The listing builds one solid part. Answer for the finished solid, in the listing's coordinates (mm). Face numbers are marked on the shaded views. Coordinates: 2 decimals unless noted, no trailing zeros. Order: outer loops, then holes, each group sorted by start corner. A loop starts at its lowest first (then second) coordinate and runs counter-clockwise, first axis right, second up. Notation, with made-up numbers: (-17.75, -36.75) -> (40.25, -36.75) arc R26 ccw to (40.25, -22.75) -> close; hole circle Ø6 at (83, 20.5). An arc over 180 degrees is marked (long way). One line per question, with ' | ' between items.
from build123d import *


# Read off the part's stored shape, not the designer's step: 抽壳1
with BuildPart() as part:
    # 草图1 → 旋转1 (revolve)
    with BuildSketch(Plane.XY, mode=Mode.PRIVATE) as revolve_1_sk:
        with BuildLine():
            Line((0, 0), (32, 0))
            Line((32, 0), (32, 2))
            Line((32, 2), (35, 2))
            Line((35, 2), (35, 5))
            Line((35, 5), (32, 5))
            Line((32, 5), (32, 7))
            Line((32, 7), (6, 12))
            Line((6, 12), (6, 15))
            ThreePointArc((6, 15), (9.486832981, 26.16227766), (0, 33))
            Line((0, 33), (0, 0))
        make_face()
    revolve(revolve_1_sk.sketch.rotate(Axis((0, 0, 0), (0, 1, 0)), 90), axis=Axis((0, 0, 0), (0, 1, 0)))

    # 抽壳1 outline → 抽壳1 (revolve, cut)
    with BuildSketch(Plane.XY):
        Polygon((29, 0), (29, 4.521953317), (0, 10.098876393), (0, 0), align=None)
    revolve(axis=Axis((0, 0, 0), (0, 1, 0)), mode=Mode.SUBTRACT)


solid = part.part
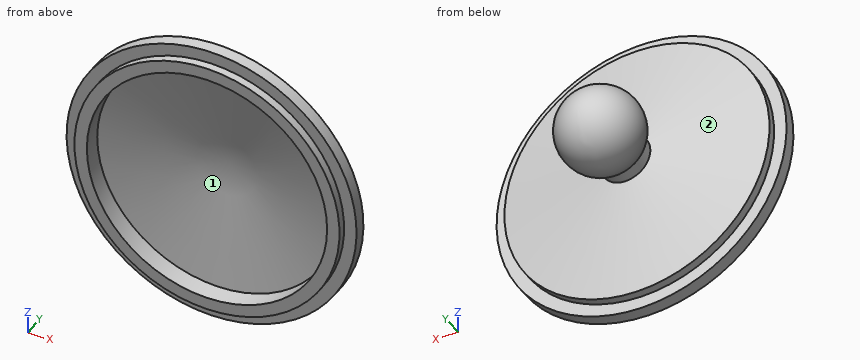
Item 1: Section B-B, the plane y = 13 is taken. Give the vertices of the cut face in (x, z).
Computed values:
outline: circle Ø12 at (0, 0)
Item 2: Determine the mould class of the marked faces 1 and 2 for opening direction X: pulls with the +X half, pulls with the -X half, needs draft (parallel to the pull), parting line crosses it, or undercut.
Computed values:
face 1: undercut | face 2: parting line crosses it
Item 3: Find the intervals of material crossed by L1, parallel to X at y = 3, z = 0; L2, parallel to X at y = 1.75, z = 0; L3, parallel to Z at x = -14.5, y = 4.5, in increasing order.
Computed values:
L1: x = -35 to -29, 29 to 35 | L2: x = -32 to -29, 29 to 32 | L3: z = -31.86 to -25.11, 25.11 to 31.86
Item 4: Each of these flat-tipped pins is pushed along its axis until it touches: pin 1 Ø1 at (y, z) = (4, -7) entering from -X; pin 2 Ø1.5 at (y, z) = (28.5, -1) entering from +X; pin 3 Ø10 at (x, z) = (21, 1.5) entering from +Y; pin 4 Ø6 at (x, z) = (27.5, -2.5) entering from -Y. Where does it stop, or does it pass through?
Computed values:
pin 1: stops at x = -34.39 | pin 2: stops at x = 8.75 | pin 3: stops at y = 10.07 | pin 4: stops at y = 0
Item 5: Section C-C, the plane y = 30 is taken. Give the vertices of the cut face in (x, z).
Computed values:
outline: circle Ø14.28 at (0, 0)
Item 6: Section A-A, the plane y = 6 is taken. Give the vertices of the cut face in (x, z), plus the area to 3 significant figures.
Computed values:
outline: circle Ø64 at (0, 0); hole circle Ø42.63 at (0, 0) | area: 1,790 mm^2
